Design review of the part built by this model. Coordinates are the model's own, in mm. A direction names the side the tool comes from. Coordinates: 2 decimals unless noted, no trailing zeros. Answer as a JSON object with one key per item and string values.
```python
from build123d import *

# Parameters (mm, degrees)
F0_R     = 11
F1_DEPTH = 3.5


with BuildPart() as f1:
    # F0 (on Top) → F1 (new body, symmetric)
    with BuildSketch(Plane.XY):
        with BuildLine():
            ThreePointArc((-5.9371989536, 9.136938762), (-4.5556948826, 8.1032503328), (-5.7171564072, 6.8272909316))
            add(Edge.make_bspline(
                [(-7.1601356012, 19.7303443127), (-9.8396121009, 17.328055376), (-11.7631082296, 12.7037080844), (-7.991697676, 6.7025448219), (-5.7171564072, 6.8272909316)],
                knots=[0, 0, 0, 0, 0.5193023993, 1, 1, 1, 1], degree=3))
            Line((-7.1601356012, 19.7303443127), (-29.2586693251, 25.4083474436))
            add(Edge.make_bspline(
                [(2.7892878075, -23.0723533458), (-9.100445471, -23.3260705726), (-26.0312299774, -19.4058078659), (-37.3351362806, -0.3188714111), (-34.0472960433, 17.7900344429), (-29.2586693251, 25.4083474436)],
                knots=[0, 0, 0, 0, 0.3603746174, 0.6556097302, 1, 1, 1, 1], degree=3))
            add(Edge.make_bspline(
                [(3.9497939315, -30), (6.3200092463, -24.0845974018), (8.4418802977, -14.4410055096), (5.618321076, -5.9348622155), (0.4188786459, -5.0226176358), (-4.661613499, -11.3368669415), (0.3789602011, -19.4366700265), (2.7892878075, -23.0723533458)],
                knots=[0, 0, 0, 0, 0.2738856545, 0.4583152945, 0.591269181, 0.7564644707, 1, 1, 1, 1], degree=3))
            add(Edge.make_bspline(
                [(24.0596541754, 29.6391923389), (31.7168351337, 22.656535609), (41.5570833778, -1.6182185805), (23.0239544155, -27.1377676606), (3.9497939315, -30)],
                knots=[0, 0, 0, 0, 0.4612146425, 1, 1, 1, 1], degree=3))
            Line((24.0596541754, 29.6391923389), (2.4210962566, 18.9946021933))
            add(Edge.make_bspline(
                [(4.6126311388, 7.1527171592), (6.9798036393, 7.6946970927), (8.5434124721, 14.7188307272), (4.6365245457, 17.2686031477), (2.4210962566, 18.9946021933)],
                knots=[0, 0, 0, 0, 0.4936475393, 1, 1, 1, 1], degree=3))
            add(Edge.make_bspline(
                [(1.2064232823, 14.5694600899), (2.7917893894, 13.7439214682), (5.0913604942, 10.1353380455), (4.6597097129, 8.3324459978), (4.6126311388, 7.1527171592)],
                knots=[0, 0, 0, 0, 0.5729073376, 1, 1, 1, 1], degree=3))
            Line((1.2064232823, 14.5694600899), (-6.7597080421, 10.5589251693))
            Line((-6.7597080421, 10.5589251693), (-5.9371989536, 9.136938762))
        make_face()
        with Locations((20.5298382789, 3.9593884721)):
            Circle(F0_R, mode=Mode.SUBTRACT)
    extrude(amount=F1_DEPTH, both=True)


solid = f1.part
```
(1) To check wall thickness, follow line 1 (X direction, y = 16.5, z = -1.5); line 2 (X direction, y = 16, z = 1.25); line 3 (Y direction, x = 12, z = 2.5). State the ranges of each line that lie inside material, in increasing order. Write a range as from..to.
Solved:
{"line 1": "x = -33.26..-9.75, 5.45..32.84", "line 2": "x = -33.41..-9.97, 5.91..33.02", "line 3": "y = -27.99..-2.99, 10.91..23.71"}
(2) Tool access review of faces 1 (the face through (-2.721, 12.592, 0.049)), 2 (the face through (-7, 0, -3.5)), 3 (the face through (-4.56, 8.13, 0.05)): name each direction out of +Z, -Z, +X, -X, +Y, -Y from which nothing blocks a thin tool from reaching the whole face with its end or side.
Solved:
{"face 1": "+Z, -Z, +Y", "face 2": "-Z, +X, -X, +Y, -Y", "face 3": "+Z, -Z"}
(3) The part is to be moulded in two halves that separate along Y. For faces 4 (the face through (-6.354, 9.858, 0.049)), 5 (the face through (-18.05, 22.53, 0.05)), 6 (the face through (-7, 0, 3.5)), say which applies: pulls with the +Y half, pulls with the -Y half, needs draft (parallel to the pull), parting line crosses it, or undercut.
Solved:
{"face 4": "undercut", "face 5": "pulls with the +Y half", "face 6": "needs draft"}
